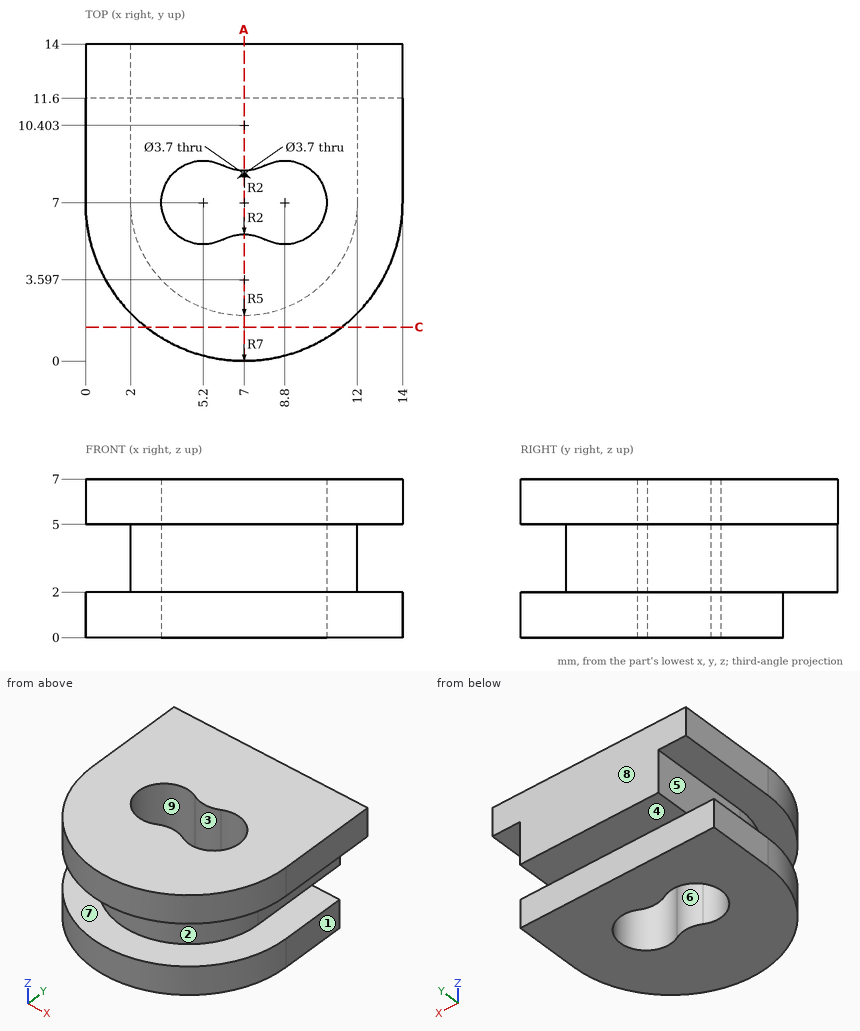
Verification items for this drawing (mm, ordinates from the low corner). A direction names the side the tool comes from. Round coordinates to 2 decimals unless told otherwise and drop trailing zeros. Order: outer loops, then holes, each group sorted by start corner. A loop starts at its lowest first (then second) coordinate and runs counter-clockwise, first axis right, second up. Notation, with made-up numbers: M 24,33 L 61,33 A21 ccw 61,59 Z; hole C -17,14.25 d3. An arc over 180 degrees is marked long. Answer in a Markdown table with one row per item. Add a question column.
Item 1: Draft check along Y on the marked faces 6, 7, 8 and 9. Enter one of: released by +Y, released by -Y, zero draft, split by the parting line, or undercut.
Item 2: Sectioned sample at A-A, the plane x = 7. Enter the section's corners in (y, z).
Item 3: Depth check by flat-ended pin: pin 1 Ø1.2 at (x, y) = (8.5, 13.5) entering from -Z; pin 2 Ø1.5 at (y, z) = (4.5, 1) entering from +X; pin 3 Ø1.5 at (y, z) = (11.5, 3) entering from -X. Enter the tip coordinate at first touch or a pass-through.
Item 4: Material ranges on L1, parallel to Z at x = 2.5, y = 2; L2, parallel to Y at x = 7, z = 1.25; L3, parallel to Y at x = 10, z = 4.5, recorded low to high. Write a range as [from, to].
Item 5: Set-up check for the marked faces 1, 2, 3, 4 and 5: record each of +Z, -Z, +X, -X, +Y, -Y from which the full face is reachable in a straight line by a thin tool's end or side.
Item 6: Sectioned sample at C-C, the plane y = 1.5. Enter the section's corners in (x, z).
Filled in:
| question | item | result |
|---|---|---|
| 1 | face 6 | undercut |
| 1 | face 7 | zero draft |
| 1 | face 8 | released by +Y |
| 1 | face 9 | undercut |
| 2 | outline | M 0,0 L 5.6,0 L 5.6,7 L 0,7 L 0,5 L 2,5 L 2,2 L 0,2 Z; M 8.4,0 L 11.6,0 L 11.6,2 L 14,2 L 14,7 L 8.4,7 Z |
| 3 | pin 1 | stops at z = 2 |
| 3 | pin 2 | stops at x = 13.78 |
| 3 | pin 3 | stops at x = 2 |
| 4 | L1 | z = [0, 2], [5, 7] |
| 4 | L2 | y = [0, 5.6], [8.4, 11.6] |
| 4 | L3 | y = [3, 5.59], [8.41, 14] |
| 5 | face 1 | +Z, -Z, +X, +Y, -Y |
| 5 | face 2 | -Y |
| 5 | face 3 | +Z, -Z |
| 5 | face 4 | -Z, +X, -X, +Y |
| 5 | face 5 | -X, +Y, -Y |
| 6 | outline | M 2.67,0 L 11.33,0 L 11.33,2 L 2.67,2 Z; M 2.67,5 L 11.33,5 L 11.33,7 L 2.67,7 Z |
